Input: part model. Units: mm. Frame: model coordinates. Face numbers are marked on the shaded views. A direction names the side the tool comes from. Round coordinates to 2 decimals unless told otherwise and drop trailing zeros. Write each loop counter-clockwise with the first axis right and the second up, starting at its lowest first coordinate (ties: lowest second). Pieces come first, ordered by that corner, then holes. Notation, with made-up numbers: (30.5, -5) -> (64.5, -5) arc R12 cw to (64.5, 16) -> close; hole circle Ø3 at (24, 49). An arc over 180 degrees is marked (long way). Write item = value, one per line.
```python
from build123d import *

# Parameters (mm, degrees)
SKETCH1_W           = 3.175
SKETCH1_H           = 28.575
BOSS_EXTRUDE1_DEPTH = 9.525
CUT_EXTRUDE1_REACH  = 19.462
SKETCH4_R           = 0.889
SKETCH5_W           = 3.175
SKETCH5_H           = 6.35
BOSS_EXTRUDE3_DEPTH = 2.54


with BuildPart() as part:
    # Sketch1 → Boss-Extrude1 (new body)
    with BuildSketch(Plane.XY):
        Rectangle(SKETCH1_W, SKETCH1_H)
    extrude(amount=BOSS_EXTRUDE1_DEPTH)

    # Sketch4 → Cut-Extrude1 (cut, up to next)
    with BuildSketch(Plane(origin=(1.5875, 0, 0), x_dir=(0, 0, -1), z_dir=(1, 0, 0)), mode=Mode.PRIVATE) as cut_extrude1_sk1:
        with Locations((-4.7625, -9.0043)):
            Circle(SKETCH4_R)
    cut_extrude1_tool1 = extrude(cut_extrude1_sk1.sketch, amount=-CUT_EXTRUDE1_REACH, mode=Mode.PRIVATE) & part.part
    # Sketch4 → Cut-Extrude1 (cut, up to next)
    with BuildSketch(Plane(origin=(1.5875, 0, 0), x_dir=(0, 0, -1), z_dir=(1, 0, 0)), mode=Mode.PRIVATE) as cut_extrude1_sk2:
        with Locations((-4.7625, 9.0043)):
            Circle(SKETCH4_R)
    cut_extrude1_tool2 = extrude(cut_extrude1_sk2.sketch, amount=-CUT_EXTRUDE1_REACH, mode=Mode.PRIVATE) & part.part
    add(cut_extrude1_tool1.solids().sort_by_distance((1.5875, -9.0043, 4.7625))[0], mode=Mode.SUBTRACT)
    add(cut_extrude1_tool2.solids().sort_by_distance((1.5875, 9.0043, 4.7625))[0], mode=Mode.SUBTRACT)

    # Sketch5 → Boss-Extrude3 (add)
    with BuildSketch(Plane.XY.offset(9.525)):
        Polygon((-1.5875, 7.9375), (-1.5875, 14.2875), (-15.875, 14.2875), (-15.875, 7.9375), (-13.335, 7.9375), align=None)
        with Locations((0, 11.1125)):
            Rectangle(SKETCH5_W, SKETCH5_H)
        Polygon((15.875, 7.9375), (15.875, 14.2875), (1.5875, 14.2875), (1.5875, 7.9375), (13.335, 7.9375), align=None)
        Polygon((15.875, 1.5875), (15.875, 7.9375), (13.335, 7.9375), (13.335, 1.809721205), align=None)
        Polygon((-13.335, 7.9375), (-15.875, 7.9375), (-15.875, 1.5875), (-13.335, 1.809721205), align=None)
    extrude(amount=BOSS_EXTRUDE3_DEPTH)


solid = part.part
```
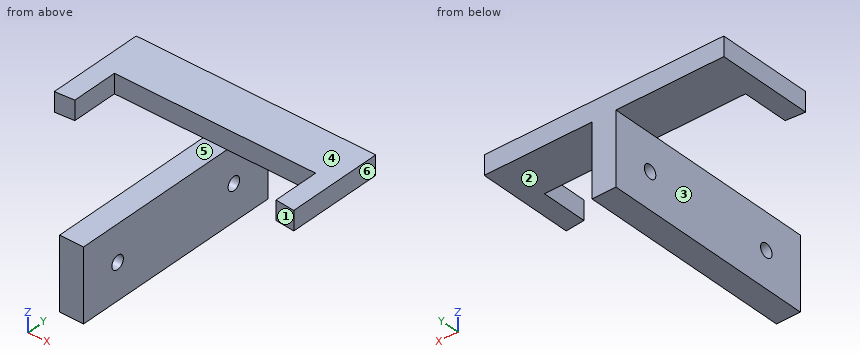
1) Access query for the marked faces 1, 2 and 3. Directions: +Z, -Z, +X, -X, +Y, -Y. A direction counts if a zero-diameter tool reaches every point of the face in a straight line with its end or side. Return the directions, or none.
Solutions:
face_1 = +Z, -Z, -Y
face_2 = -Z, +X, +Y, -Y
face_3 = -Z, -X, +Y, -Y
2) Cut plane A-A (y = 7). Return the cut outline in (x, z) (1 decimal), and give its area (3 significant figures).
Solutions:
outline = (-15.9, 9.5) -> (-13.3, 9.5) -> (-13.3, 12.1) -> (-15.9, 12.1) -> close; (-1.6, 0) -> (1.6, 0) -> (1.6, 9.5) -> (-1.6, 9.5) -> close; (13.3, 9.5) -> (15.9, 9.5) -> (15.9, 12.1) -> (13.3, 12.1) -> close
area = 43.1 mm^2
3) Cut plane D-D (z = 11.25). Return the cut outline in (x, y) (1 decimal), and give its area (3 significant figures).
Solutions:
outline = (-15.9, 1.6) -> (-13.3, 1.8) -> (-13.3, 7.9) -> (13.3, 7.9) -> (13.3, 1.8) -> (15.9, 1.6) -> (15.9, 14.3) -> (-15.9, 14.3) -> close
area = 233 mm^2
4) Cut plane B-B (z = 4.25). Return the cut outline in (x, y), and give its area (3 significant figures).
Solutions:
outline = (-1.59, -14.29) -> (1.59, -14.29) -> (1.59, -9.73) -> (-1.59, -9.73) -> close; (-1.59, -8.28) -> (1.59, -8.28) -> (1.59, 8.28) -> (-1.59, 8.28) -> close; (-1.59, 9.73) -> (1.59, 9.73) -> (1.59, 14.29) -> (-1.59, 14.29) -> close
area = 81.5 mm^2
5) First-contact query: P1, Ø6, axis at x = -3, y = 8.5, coming from the -Z side; P2, Ø14, axis at x = -10, y = 5.5, coming from the -Z side (3 decimals); P3, Ø2.5, axis at y = -9, z = 4.76, coming from the -X side; P4, Ø0.8, axis at x = -6.5, z = 10.5, coming from the -Y side. Flat tips, straight axial feed; report the tip coordinate or a pass-through.
Solutions:
P1 = 0
P2 = 9.525
P3 = -1.59
P4 = 7.94
6) Cut plane C-C (x = 0). Return the cut outline in (y, z) (1 decimal).
Solutions:
outline = (-14.3, 0) -> (14.3, 0) -> (14.3, 12.1) -> (7.9, 12.1) -> (7.9, 9.5) -> (-14.3, 9.5) -> close; hole circle Ø1.8 at (-9, 4.8); hole circle Ø1.8 at (9, 4.8)
7) Draft query along X for the marked faces 4, 5 and 6. Return one class per face: +X half, -X half, draft (parallel to the pull), parting line (faces both ways), or undercut.
Solutions:
face_4 = draft
face_5 = undercut
face_6 = +X half
8) Line query: L1, parallel to X at y = -3.5, z = 1.25; L2, parallel to X at y = 7.5, z = 10.25 (3 decimals); L3, parallel to Y at x = -3, z = 10.75. Output: solid intervals per line, ascending. Write a range as from..to.
Solutions:
L1 = -1.59..1.59
L2 = -15.875..-13.335, 13.335..15.875
L3 = 7.94..14.29
